Check sheet for the modelled part. Datum: model origin and axes. Units: mm. A direction names the side the tool comes from. Round coordinates to 2 decimals unless told otherwise and drop trailing zeros. Order: outer loops, then holes, each group sorted by start corner. A loop starts at its lowest first (then second) coordinate and runs counter-clockwise, first axis right, second up. Notation, with made-up numbers: M 10.5,-8 L 53.5,-8 A17 cw 53.5,6 Z; hole C 75,-3.5 d9. An arc over 180 degrees is marked long. One line per item, written item: value. Start each with the question number.
(1) Release check for a two-part mould opening along Z. For faces 1 (the face through (0, 36.3, 16.9)), 2 (the face through (-18.13, -20.46, 11.94)), 3 (the face through (2.52, 42.88, 15.54)), 4 (the face through (-23, -5.814, 5)) record: released by +Z, released by -Z, zero draft, split by the parting line, or undercut.
(2) Cross-section at D-D, the plane z = 6. Enter the section's corners in (x, y) (1 decimal), and give its area (3 significant figures).
(3) Depth check by flat-ended pin: pin 1 Ø10 at (y, z) = (25.5, 30) entering from -X; pin 2 Ø4.5 at (y, z) = (-10, 4) entering from -X; pin 3 Ø6 at (x, y) = (-0.5, 15) entering from -Z. Enter the tip coordinate at first touch or a pass-through.
(4) Cross-section at C-C, the plane z = 24. Enter the section's corners in (x, y).
(5) Access from +Z, -Z, +X, -X, +Y, -Y to the whole of each face (thin tool, end or side, straight path). Record for faces 5 (the face through (-2.52, -42.88, 15.54)), 6 (the face through (19.7, -9, 5)).
(6) Thickness scan on L1, parallel to Y at x = 10, z = 5; L2, parallel to Y at x = -15, z = 3.5; L3, parallel to X at y = 17, z = 2.5. Record the ranges inside material, lowest first.
from build123d import *

# Parameters (mm, degrees)
F0_W        = 101.6
F0_H        = 101.6
F1_DEPTH    = 34.925
F2_T1_DEPTH = 299.3404177556
F2_T3_DEPTH = 299.3404177556
F3_R        = 3.175
F4_DEPTH    = 12.7
F5_R        = 3.175
F6_DEPTH    = 12.7
F7_R        = 3.175
F8_DEPTH    = 12.7
F9_R        = 3.175
F10_DEPTH   = 12.7
F11_W       = 75.6562831473
F11_H       = 25.4
F12_DEPTH   = 25.4
F13_SIZE2   = 25.39999
F13_SIZE    = 2.53999
F15_DEPTH   = 12.7
F16_R       = 2.54


# Not quite as in the source:
# - a fillet or chamfer that OpenCascade refuses, or shapes differently, is made with other operations: its cross-section is extruded or revolved along the edge and cut away or added
# - a fillet or chamfer is up to 0.001 mm smaller than in the source, because OpenCascade refuses the exact size


with BuildPart() as f1:
    # F0 (on Top) → F1 (new body)
    with BuildSketch(Plane.XY):
        Rectangle(F0_W, F0_H)
    extrude(amount=F1_DEPTH)

    # F2: chamfer of 3.3274 x 38.0323560322 on 4 edges, made by hand

    # F2_s2 → F2_t1 (cut)
    with BuildSketch(Plane.XZ.offset(-149.6702088778)):
        Polygon((-50.8, -3.1073560322), (-47.4726, 34.925), (-50.8, 34.925), align=None)
        Polygon((50.8, -3.1073560322), (47.4726, 34.925), (50.8, 34.925), align=None)
    extrude(amount=F2_T1_DEPTH, mode=Mode.SUBTRACT)

    # F2_s4 → F2_t3 (cut)
    with BuildSketch(Plane.YZ.offset(-149.6702088778)):
        Polygon((-50.8, -3.1073560322), (-47.4726, 34.925), (-50.8, 34.925), align=None)
        Polygon((50.8, -3.1073560322), (47.4726, 34.925), (50.8, 34.925), align=None)
    extrude(amount=F2_T3_DEPTH, mode=Mode.SUBTRACT)

    # F3 (on face) → F4 (cut)
    with BuildSketch(Plane(origin=(0, 50.1443235703, 4.3870598526), x_dir=(-1, 0, 0), z_dir=(0, 0.9961946981, 0.0871557427))):
        with Locations((0, 13.6719250414)):
            Circle(F3_R)
    extrude(amount=-F4_DEPTH, mode=Mode.SUBTRACT)

    # F5 (on face) → F6 (cut)
    with BuildSketch(Plane(origin=(0, -50.1443235703, 4.3870598526), x_dir=(1, 0, 0), z_dir=(0, -0.9961946981, 0.0871557427))):
        with Locations((0, 13.6719250414)):
            Circle(F5_R)
    extrude(amount=-F6_DEPTH, mode=Mode.SUBTRACT)

    # F7 (on face) → F8 (cut)
    with BuildSketch(Plane(origin=(50.1443235703, 0, 4.3870598526), x_dir=(0, 1, 0), z_dir=(0.9961946981, 0, 0.0871557427))):
        with Locations((0, 13.6719250414)):
            Circle(F7_R)
    extrude(amount=-F8_DEPTH, mode=Mode.SUBTRACT)

    # F9 (on face) → F10 (cut)
    with BuildSketch(Plane(origin=(-50.1443235703, 0, 4.3870598526), x_dir=(0, -1, 0), z_dir=(-0.9961946981, 0, 0.0871557427))):
        with Locations((0, 13.6719250414)):
            Circle(F9_R)
    extrude(amount=-F10_DEPTH, mode=Mode.SUBTRACT)

    # F11 (on face) → F12 (cut)
    with BuildSketch(Plane(origin=(0, 0, 0), x_dir=(1, 0, 0), z_dir=(0, 0, -1))):
        with Locations((0, -18.7781415736)):
            Rectangle(F11_W, F11_H)
    extrude(amount=-F12_DEPTH, mode=Mode.SUBTRACT)

    # F13 (size 2.54 and 25.4 in the source; OpenCascade refuses exactly that, so slightly less here)
    f13_edges = [f1.edges().sort_by_distance(p)[0] for p in [
        (0, 6.078142, 25.4),
        (-37.828142, 18.778142, 25.4),
        (0, 31.478142, 25.4),
        (37.828142, 18.778142, 25.4),
    ]]
    f13_side = f1.faces().sort_by_distance((0, 18.778142, 25.4))[0]
    chamfer(f13_edges, length=F13_SIZE, length2=F13_SIZE2, reference=f13_side)

    # F14 (on face) → F15 (cut)
    with BuildSketch(Plane(origin=(0, 0, 0), x_dir=(1, 0, 0), z_dir=(0, 0, -1))):
        with BuildLine():
            Line((-19.6998585016, 11.6611556837), (-10.5549017823, 11.6611556837))
            ThreePointArc((-10.5549017823, 11.6611556837), (-5.7924017823, 16.4236556837), (-10.5549017823, 21.1861556837))
            Line((-10.5549017823, 21.1861556837), (-19.6998585016, 21.1861556837))
            Line((-19.6998585016, 21.1861556837), (-25.4897605628, 21.1861556837))
            Line((-25.4897605628, 21.1861556837), (-25.4897605628, 11.6611556837))
            Line((-25.4897605628, 11.6611556837), (-25.4897605628, 5.814129021))
            Line((-25.4897605628, 5.814129021), (-19.6998585016, 5.814129021))
            Line((-19.6998585016, 5.814129021), (-19.6998585016, 11.6611556837))
        make_face()
        with BuildLine():
            Line((25.4897605628, 11.6611556837), (25.4897605628, 21.1861556837))
            Line((25.4897605628, 21.1861556837), (19.6998585016, 21.1861556837))
            Line((19.6998585016, 21.1861556837), (10.5549017823, 21.1861556837))
            ThreePointArc((10.5549017823, 21.1861556837), (5.7924017823, 16.4236556837), (10.5549017823, 11.6611556837))
            Line((10.5549017823, 11.6611556837), (19.6998585016, 11.6611556837))
            Line((19.6998585016, 11.6611556837), (19.6998585016, 5.814129021))
            Line((19.6998585016, 5.814129021), (25.4897605628, 5.814129021))
            Line((25.4897605628, 5.814129021), (25.4897605628, 11.6611556837))
        make_face()
    extrude(amount=-F15_DEPTH, mode=Mode.SUBTRACT)

    # F16
    f16_edges = [f1.edges().sort_by_distance(p)[0] for p in [
        (-15.12738, -11.661156, 12.7),
        (-5.792402, -16.423656, 12.7),
        (-18.022331, -21.186156, 12.7),
        (-25.489761, -13.500142, 12.7),
        (-22.59481, -5.814129, 12.7),
        (-19.699859, -8.737642, 12.7),
        (18.022331, -21.186156, 12.7),
        (5.792402, -16.423656, 12.7),
        (15.12738, -11.661156, 12.7),
        (19.699859, -8.737642, 12.7),
        (22.59481, -5.814129, 12.7),
        (25.489761, -13.500142, 12.7),
    ]]
    fillet(f16_edges, radius=F16_R)


solid = f1.part
Values found:
1. face 1: undercut
1. face 2: released by -Z
1. face 3: undercut
1. face 4: zero draft
2. outline: M -50,-50 L 50,-50 L 50,50 L -50,50 Z; hole M -37.2,6.7 L 37.2,6.7 L 37.2,30.9 L -37.2,30.9 Z; hole M -25.5,-21.2 L -10.6,-21.2 A4.8 ccw -10.6,-11.7 L -19.7,-11.7 L -19.7,-5.8 L -25.5,-5.8 Z; hole M 10.6,-21.2 L 25.5,-21.2 L 25.5,-5.8 L 19.7,-5.8 L 19.7,-11.7 L 10.6,-11.7 A4.8 ccw Z
2. area: 7,780 mm^2
3. pin 1: x = -48.34
3. pin 2: x = -50.38
3. pin 3: z = 25.4
4. outline: M -48.43,-48.43 L 48.43,-48.43 L 48.43,48.43 L -48.43,48.43 Z; hole M -35.43,8.48 L 35.43,8.48 L 35.43,29.08 L -35.43,29.08 Z
5. face 5: none
5. face 6: -Z
6. L1: -50.09 to -21.15, -11.69 to 6.58, 30.98 to 50.09
6. L2: -50.22 to -21.19, -11.66 to 6.43, 31.13 to 50.22
6. L3: -50.31 to -37.58, 37.58 to 50.31
